```python
from build123d import *

# Parameters (mm, degrees)
F0_W        = 12.7
F0_H        = 12.7
F1_DEPTH    = 25.4
F2_T1_DEPTH = 69.85
F3_R        = 5.08


# Not quite as in the source:
# - a fillet or chamfer that OpenCascade refuses, or shapes differently, is made with other operations: its cross-section is extruded or revolved along the edge and cut away or added


with BuildPart() as f1:
    # F0 (on Front) → F1 (new body)
    with BuildSketch(Plane.XZ):
        Polygon((12.7, 0), (0, 0), (-12.7, 0), (-25.4, 0), (-38.1, 0), (-50.8, 0), (-63.5, 0), (-76.2, 0), (-76.2, -12.7), (0, -12.7), (76.2, -12.7), (76.2, 0), (63.5, 0), (50.8, 0), (38.1, 0), (25.4, 0), align=None)
        with Locations((-6.35, 6.35)):
            Rectangle(F0_W, F0_H)
        with Locations((19.05, 6.35)):
            Rectangle(F0_W, F0_H)
        with Locations((-31.75, 6.35)):
            Rectangle(F0_W, F0_H)
        with Locations((44.45, 6.35)):
            Rectangle(F0_W, F0_H)
        with Locations((-57.15, 6.35)):
            Rectangle(F0_W, F0_H)
        with Locations((69.85, 6.35)):
            Rectangle(F0_W, F0_H)
    extrude(amount=F1_DEPTH)

    # F2: fillet of radius 8.89 on 12 edges, made by hand

    # F2_s2 → F2_t1 (cut)
    with BuildSketch(Plane.XZ.offset(-22.225)):
        with BuildLine():
            ThreePointArc((-54.61, 12.7), (-60.8961792847, 10.0961792847), (-63.5, 3.81))
            Line((-63.5, 3.81), (-63.5, 12.7))
            Line((-63.5, 12.7), (-54.61, 12.7))
        make_face()
        with BuildLine():
            ThreePointArc((-50.8, 3.81), (-53.4038207153, 10.0961792847), (-59.69, 12.7))
            Line((-59.69, 12.7), (-50.8, 12.7))
            Line((-50.8, 12.7), (-50.8, 3.81))
        make_face()
        with BuildLine():
            ThreePointArc((-29.21, 12.7), (-35.4961792847, 10.0961792847), (-38.1, 3.81))
            Line((-38.1, 3.81), (-38.1, 12.7))
            Line((-38.1, 12.7), (-29.21, 12.7))
        make_face()
        with BuildLine():
            ThreePointArc((-25.4, 3.81), (-28.0038207153, 10.0961792847), (-34.29, 12.7))
            Line((-34.29, 12.7), (-25.4, 12.7))
            Line((-25.4, 12.7), (-25.4, 3.81))
        make_face()
        with BuildLine():
            ThreePointArc((-3.81, 12.7), (-10.0961792847, 10.0961792847), (-12.7, 3.81))
            Line((-12.7, 3.81), (-12.7, 12.7))
            Line((-12.7, 12.7), (-3.81, 12.7))
        make_face()
        with BuildLine():
            ThreePointArc((0, 3.81), (-2.6038207153, 10.0961792847), (-8.89, 12.7))
            Line((-8.89, 12.7), (0, 12.7))
            Line((0, 12.7), (0, 3.81))
        make_face()
        with BuildLine():
            ThreePointArc((21.59, 12.7), (15.3038207153, 10.0961792847), (12.7, 3.81))
            Line((12.7, 3.81), (12.7, 12.7))
            Line((12.7, 12.7), (21.59, 12.7))
        make_face()
        with BuildLine():
            ThreePointArc((25.4, 3.81), (22.7961792847, 10.0961792847), (16.51, 12.7))
            Line((16.51, 12.7), (25.4, 12.7))
            Line((25.4, 12.7), (25.4, 3.81))
        make_face()
        with BuildLine():
            ThreePointArc((46.99, 12.7), (40.7038207153, 10.0961792847), (38.1, 3.81))
            Line((38.1, 3.81), (38.1, 12.7))
            Line((38.1, 12.7), (46.99, 12.7))
        make_face()
        with BuildLine():
            ThreePointArc((50.8, 3.81), (48.1961792847, 10.0961792847), (41.91, 12.7))
            Line((41.91, 12.7), (50.8, 12.7))
            Line((50.8, 12.7), (50.8, 3.81))
        make_face()
        with BuildLine():
            ThreePointArc((76.2, 3.81), (73.5961792847, 10.0961792847), (67.31, 12.7))
            Line((67.31, 12.7), (76.2, 12.7))
            Line((76.2, 12.7), (76.2, 3.81))
        make_face()
        with BuildLine():
            ThreePointArc((72.39, 12.7), (66.1038207153, 10.0961792847), (63.5, 3.81))
            Line((63.5, 3.81), (63.5, 12.7))
            Line((63.5, 12.7), (72.39, 12.7))
        make_face()
    extrude(amount=F2_T1_DEPTH, mode=Mode.SUBTRACT)

    # F3
    f3_edges = [f1.edges().sort_by_distance(p)[0] for p in [
        (-63.5, -12.7, 0),
        (-50.8, -12.7, 0),
        (-38.1, -12.7, 0),
        (-25.4, -12.7, 0),
        (-12.7, -12.7, 0),
        (0, -12.7, 0),
        (12.7, -12.7, 0),
        (38.1, -12.7, 0),
        (63.5, -12.7, 0),
        (50.8, -12.7, 0),
        (25.4, -12.7, 0),
    ]]
    fillet(f3_edges, radius=F3_R)


solid = f1.part
```
Here's how the part is built. I have some questions about the finished solid (model axes, mm). A direction names the side the tool comes from. Give positions to 0.01 mm unless a question says otherwise; leave off trailing zeros. Loops run counter-clockwise (first coordinate to the right, second up) from the corner with the lowest first, then second, coordinate; pieces in that order, holes last. Notation, with made-up numbers: M -16.5,69.5 L 22.5,69.5 A21 ccw 22.5,80.5 Z; hole C 24,-24.5 d9. An arc over 180 degrees is marked long. Use one line per item in the form item = value. Start each with the question number.
Q1. Will these pins go through, and if not, where does the flat tip stop? pin 1 Ø2 at (x, y) = (-44, -15.5) entering from +Z; pin 2 Ø8.5 at (x, y) = (-71.5, -12) entering from +Z.
Q2. If we section it at A-A (z = 9.75): Write out the boundary of the cut face in (x, y).
Q3. If we section it at C-C (x = 48): Write out the boundary of the cut face in (y, z), then the cut area to 3 significant figures.
Q4. Thinking about a two-plate mould opening in X: for faces 4 (the cylindrical face through (23.44, -12.52, 9.38)), 5 (the cylindrical face through (-61.44, -12.52, 9.5)), 6 (the flat face through (76.2, -13, -5)), 7 (the flat face through (-1, -13, -12.7)), which applies, +X half, -X half, draft (parallel to the pull), parting line (faces both ways), or undercut?
Q5. If we section it at B-B (x = -58.5): Write out the boundary of the cut face in (y, z).
Q6. I need wall thicknesses on line 1 along X through (y, z) = (-10.75, 4); line 2 along X through (y, z) = (-17.75, 9.5); line 3 along Z through (x, y) = (19, -24). Which ranges of each line are inside material? Lowest first, please.
Q7. Which directions (+Z, -Z, +X, -X, +Y, -Y) give clear straight access to the entire face, cutting with the end or side of a thin tool? Please do faces 1 (the cylindrical face through (-36.04, -12.52, 9.5)), 2 (the flat face through (-72, -13, 0)), 3 (the cylindrical face through (74.485, -12.522, 9.059)).
Taken from the geometry:
q1.pin_1 = 0
q1.pin_2 = 0.16
q2.outline = M -61.22,-25.4 L -53.08,-25.4 L -53.08,0 L -61.22,0 Z; M -35.82,-25.4 L -27.68,-25.4 L -27.68,0 L -35.82,0 Z; M -10.42,-25.4 L -2.28,-25.4 L -2.28,0 L -10.42,0 Z; M 14.98,-25.4 L 23.12,-25.4 L 23.12,0 L 14.98,0 Z; M 40.38,-25.4 L 48.52,-25.4 L 48.52,0 L 40.38,0 Z; M 65.78,-25.4 L 73.92,-25.4 L 73.92,0 L 65.78,0 Z
q3.outline = M -25.4,-12.7 L 0,-12.7 L 0,10.29 L -25.4,10.29 Z
q3.area = 584 mm^2
q4.face_4 = undercut
q4.face_5 = -X half
q4.face_6 = +X half
q4.face_7 = draft
q5.outline = M -25.4,-12.7 L 0,-12.7 L 0,11.8 L -25.4,11.8 Z
q6.line_1 = -63.56 to -50.74, -38.16 to -25.34, -12.76 to 0.06, 12.64 to 25.46, 38.04 to 50.86, 63.44 to 76.2
q6.line_2 = -61.44 to -52.86, -36.04 to -27.46, -10.64 to -2.06, 14.76 to 23.34, 40.16 to 48.74, 65.56 to 74.14
q6.line_3 = -12.7 to 12.31
q7.face_1 = +Z, +Y, -Y
q7.face_2 = +Z, -X, +Y, -Y
q7.face_3 = +Z, +X, +Y, -Y
